Build history of the part. All positions in model axes, mm. A direction names the side the tool comes from. Give positions to 0.01 mm unless a question says otherwise; leave off trailing zeros. Write each loop counter-clockwise with the first axis right and the second up, starting at its lowest first coordinate (ties: lowest second). Pieces come first, ordered by that corner, then holes. Notation, with made-up numbers: (-35, 42) - (19, 42) arc R28 ccw to (19, 60) - close; hole circle Ø6 at (12.25, -31.75). An arc over 180 degrees is marked (long way). Use one line per item in the form item = value. Start each with the question number.
from build123d import *

# Parameters (mm, degrees)
F1_DEPTH = 35.940009
F2_T     = -2.38125
F3_W     = 19.757492
F3_H     = 31.177509
F4_DEPTH = 2.38125
F5_W     = 2.38125
F5_H     = 8.17333
F5_W_2   = 8.17333
F5_H_2   = 2.38125
F6_DEPTH = 1.5875


with BuildPart() as f1:
    # F0 (on Top) → F1 (new body)
    with BuildSketch(Plane.XY):
        with BuildLine():
            ThreePointArc((27.694992, -27.694992), (19.583316, -8.111675), (0, 0))
            Line((0, 0), (-2.54, 0))
            Line((-2.54, 0), (-2.54, -24.519992))
            Line((-2.54, -24.519992), (0, -24.519992))
            ThreePointArc((0, -24.519992), (2.245064, -25.449928), (3.175, -27.694992))
            Line((3.175, -27.694992), (3.175, -36.909985))
            Line((3.175, -36.909985), (27.694992, -36.909985))
            Line((27.694992, -36.909985), (27.694992, -27.694992))
        make_face()
    extrude(amount=F1_DEPTH)

    # F2
    f2_openings = [f1.faces().sort_by_distance(p)[0] for p in [
        (-2.54, -12.259996, 17.970005),
    ]]
    offset(amount=F2_T, openings=f2_openings)

    # F3 (on face) → F4 (cut)
    with BuildSketch(Plane.XZ.offset(36.909985)):
        with Locations((15.434996, 17.970005)):
            Rectangle(F3_W, F3_H)
    extrude(amount=-F4_DEPTH, mode=Mode.SUBTRACT)

    # F5 (on face) → F6 (join)
    with BuildSketch(Plane.XY.offset(35.940009)):
        with Locations((1.190625, -12.259996)):
            Rectangle(F5_W, F5_H)
        with Locations((15.434996, -33.17936)):
            Rectangle(F5_W_2, F5_H_2)
    extrude(amount=F6_DEPTH)


solid = f1.part
(1) Cut at C-C, the plane x = 4. Give the cut face in (y, z).
(2) Cut at D-D, the plane y = -17. Give the cut face in (x, z).
(3) Two-plate mould, pull along Z, no slides. Class faces 6 (the flat face through (-2.54, -23, 18)), 7 (the flat face through (12, -18, 0)), 8 (the flat face through (-1, -22.139, 18)): +Z half, -Z half, draft (parallel to the pull), parting line (faces both ways), or undercut.
(4) Wall check: line 1 (X direction, y = -31, z = 27.5) (3 decimals); line 2 (Z direction, x = 16, y = -8.5); line 3 (Z direction, x = 3.5, y = -2.5). Give the ranges that are in metal, low to high. Write a range as from..to.
(5) Pin check, flat tips, straight feed: pin 1 Ø0.5 at (x, z) = (1.5, 36.5) entering from +Y; pin 2 Ø8 at (x, z) = (15, 26) entering from +Y; pin 3 Ø14 at (x, y) = (13, -15.5) entering from +Z. Stop position of each tip, or through.
(6) Cut at B-B, the plane y = -26.5. Give the cut face in (x, z).
(7) Which spindle directions (+Z, -Z, +X, -X, +Y, -Y) get a long thin tool onto all of the face, cutting with end or side? Do faces 1 (the flat face through (11.348, -33, 37)), 2 (the flat face through (3.175, -32, 18)), 3 (the flat face through (15, -34.37, 37)), 4 (the flat face through (19.522, -33, 37)), 5 (the flat face through (25.314, -32, 18)). Say none if no direction does.
Solution:
q1.outline = (-36.91, 0) - (-0.29, 0) - (-0.29, 35.94) - (-36.91, 35.94) - close; hole (-23.84, 2.38) - (-2.7, 2.38) - (-2.7, 33.56) - (-23.84, 33.56) - close
q2.outline = (-2.54, 0) - (25.55, 0) - (25.55, 35.94) - (-2.54, 35.94) - (-2.54, 33.56) - (22.94, 33.56) - (22.94, 2.38) - (-2.54, 2.38) - close
q3.face_6 = draft
q3.face_7 = -Z half
q3.face_8 = undercut
q4.line_1 = 3.175..5.556, 25.314..27.695
q4.line_2 = 0..2.38, 33.56..35.94
q4.line_3 = 0..35.94
q5.pin_1 = -8.17
q5.pin_2 = -2.28
q5.pin_3 = 35.94
q6.outline = (2.94, 0) - (27.67, 0) - (27.67, 35.94) - (2.94, 35.94) - close; hole (5.43, 2.38) - (25.29, 2.38) - (25.29, 33.56) - (5.43, 33.56) - close
q7.face_1 = +Z, -X, +Y, -Y
q7.face_2 = +Z, -Z, -X, -Y
q7.face_3 = +Z, +X, -X, -Y
q7.face_4 = +Z, +X, +Y, -Y
q7.face_5 = -Y
